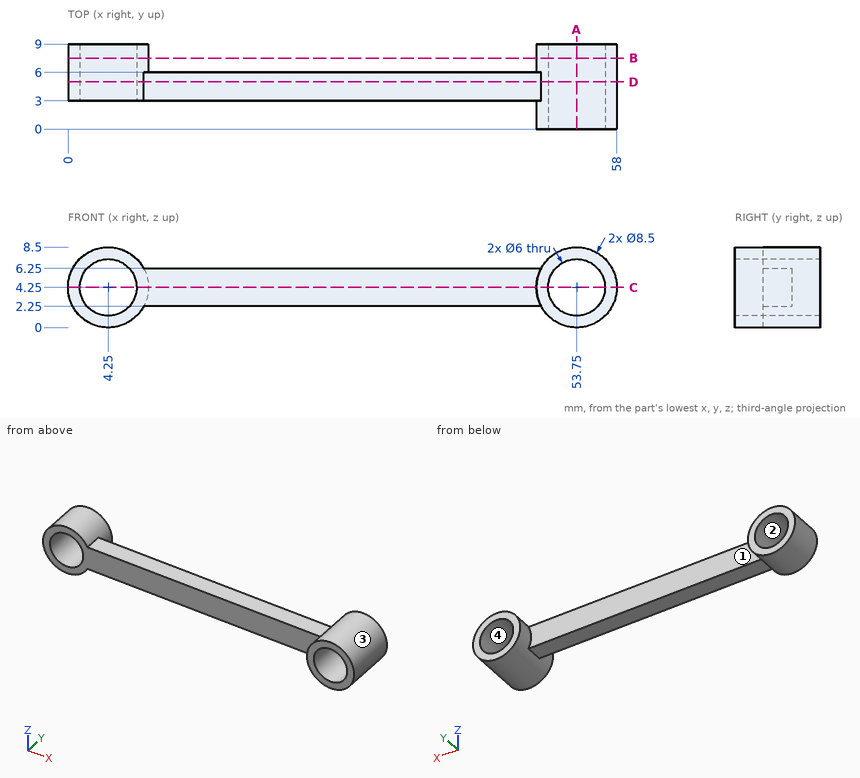
Could you check a few things on this drawing? It's one solid part, dimensions in mm from its lowest x, y, z. Round coordinates to 2 decimals unless told otherwise and drop trailing zeros. Order: outer loops, then holes, each group sorted by start corner. A loop starts at its lowest first (then second) coordinate and runs counter-clockwise, first axis right, second up.
Q1. Imagine slicing it at A-A, the plane x = 53.75. List the corners of the cut face in (y, z) for me.
Geometry says:
outline: (0, 0) - (9, 0) - (9, 1.25) - (0, 1.25) - close; (0, 7.25) - (9, 7.25) - (9, 8.5) - (0, 8.5) - close
Q2. Imagine slicing it at C-C, the plane z = 4.25. List the corners of the cut face in (x, y) for me, then the cut area to 4 significant figures.
Geometry says:
outline: (0, 3) - (1.25, 3) - (1.25, 9) - (0, 9) - close; (7.25, 3) - (49.5, 3) - (49.5, 0) - (50.75, 0) - (50.75, 9) - (49.5, 9) - (49.5, 6) - (8.5, 6) - (8.5, 9) - (7.25, 9) - close; (56.75, 0) - (58, 0) - (58, 9) - (56.75, 9) - close
area: 160.5 mm2
Q3. Imagine slicing it at D-D, the plane y = 5. List the corners of the cut face in (x, z) for me, then the cut area to 3 significant figures.
Geometry says:
outline: (8, 2.25) - (50, 2.25) arc R4.25 ccw (long way) to (50, 6.25) - (8, 6.25) arc R4.25 ccw (long way) to start; hole circle Ø6 at (4.25, 4.25); hole circle Ø6 at (53.75, 4.25)
area: 222 mm2
Q4. Please list where these lines run through material, in increasing order: probe 1 along X at (y, z) = (6.5, 4.5); probe 2 along X at (y, z) = (4.5, 4.25); probe 3 along X at (y, z) = (2, 4.25).
Geometry says:
probe 1: x = 0.01 to 1.26, 7.24 to 8.49, 49.51 to 50.76, 56.74 to 57.99
probe 2: x = 0 to 1.25, 7.25 to 50.75, 56.75 to 58
probe 3: x = 49.5 to 50.75, 56.75 to 58
Q5. Thinking about a two-plate mould opening in Z: for the marked faces 1, 2, 3 and 4, which applies, released by +Z, released by -Z, zero draft, split by the parting line, or undercut?
Geometry says:
face 1: zero draft
face 2: undercut
face 3: split by the parting line
face 4: undercut
Q6. Imagine slicing it at B-B, the plane y = 7.5. List the corners of the cut face in (x, z) for me, then the cut area to 3 significant figures.
Geometry says:
outline: circle Ø8.5 at (4.25, 4.25); circle Ø8.5 at (53.75, 4.25); hole circle Ø6 at (4.25, 4.25); hole circle Ø6 at (53.75, 4.25)
area: 56.9 mm2
Q7. I'm going to push flat-ended pins straight in: P1, Ø1, axis at y = 5, z = 2, coming from the -X side; P2, Ø2, axis at x = 41.5, y = 4, coming from the -Z side; P3, Ø4, axis at x = 21.5, z = 6.5, coming from the -Y side. Where does each tip first touch, or does it pass through?
Geometry says:
P1: stops at x = 0.38
P2: stops at z = 2.25
P3: stops at y = 3
